```python
from build123d import *
from build123d.topology import SkipClean

# Parameters (mm, degrees)
CROQUIS1_R                 = 18
SALIENTE_EXTRUIR1_DEPTH    = 3.5
SALIENTE_EXTRUIR5_DEPTH    = 3.27
CORTAR_EXTRUIR4_REACH      = 62.83
CORTAR_EXTRUIR4_END_RADIUS = 18
CROQUIS5_W                 = 14
CROQUIS5_H                 = 0.27
CORTAR_EXTRUIR2_DEPTH      = 21
CORTAR_EXTRUIR5_DEPTH      = 10
SALIENTE_EXTRUIR6_START    = -2.2
SALIENTE_EXTRUIR6_DEPTH    = 2.2
CORTAR_EXTRUIR8_START      = 0.27
CROQUIS8_R                 = 18
CORTAR_EXTRUIR8_DEPTH      = 0.27
SALIENTE_EXTRUIR7_START    = 2.47
SALIENTE_EXTRUIR7_DEPTH    = 2.47
SALIENTE_EXTRUIR9_DEPTH    = 10
CORTAR_EXTRUIR9_START      = 10
CORTAR_EXTRUIR9_DEPTH      = 10
CROQUIS13_W                = 12.6
CROQUIS13_H                = 4.84
CROQUIS13_H_2              = 4.65
SALIENTE_EXTRUIR10_DEPTH   = 4
CROQUIS12_R                = 1
CORTAR_EXTRUIR10_DEPTH     = 18.85


with BuildPart() as part:
    # Croquis1 → Saliente-Extruir1 (new body)
    with BuildSketch(Plane.XY):
        Circle(CROQUIS1_R)
    extrude(amount=SALIENTE_EXTRUIR1_DEPTH)

    # Croquis2 → Saliente-Extruir5 (add)
    with BuildSketch(Plane.XY):
        with BuildLine():
            Line((4, 39.111635425), (4, 20.615528128))
            ThreePointArc((4, 20.615528128), (5.515132245, 20.262855582), (7, 19.798989873))
            Line((7, 19.798989873), (7, 39.928035252))
            Line((7, 39.928035252), (4, 39.928035252))
            Line((4, 39.928035252), (4, 39.111635425))
        make_face()
        with BuildLine():
            Line((-4, 20.615528128), (-4, 17.549928775))
            ThreePointArc((-4, 17.549928775), (0, 18), (4, 17.549928775))
            Line((4, 17.549928775), (4, 20.615528128))
            ThreePointArc((4, 20.615528128), (0, 21), (-4, 20.615528128))
        make_face()
        with BuildLine():
            Line((-4, 39.111635425), (-4, 20.615528128))
            ThreePointArc((-4, 20.615528128), (0, 21), (4, 20.615528128))
            Line((4, 20.615528128), (4, 39.111635425))
            Line((4, 39.111635425), (4, 39.928035252))
            Line((4, 39.928035252), (-4, 39.928035252))
            Line((-4, 39.928035252), (-4, 39.111635425))
        make_face()
        with BuildLine():
            ThreePointArc((-7, 19.798989873), (-5.515132245, 20.262855582), (-4, 20.615528128))
            Line((-4, 20.615528128), (-4, 39.111635425))
            Line((-4, 39.111635425), (-4, 39.928035252))
            Line((-4, 39.928035252), (-7, 39.928035252))
            Line((-7, 39.928035252), (-7, 19.798989873))
        make_face()
    extrude(amount=SALIENTE_EXTRUIR5_DEPTH)

    # Cortar-Extruir4: up to this cylinder (the profile starts outside it)
    with SkipClean():  # the faces are left unmerged after this step: merging them gives an invalid solid
        cortar_extruir4_end = Plane(origin=(0, 0, 0.135), z_dir=(0, 0, -1)) * Cylinder(CORTAR_EXTRUIR4_END_RADIUS, 162.66, mode=Mode.PRIVATE)
        # Croquis5 → Cortar-Extruir4 (cut, up to the surface)
        with BuildSketch(Plane(origin=(0, 40, 0), x_dir=(1, 0, 0), z_dir=(0, 1, 0)), mode=Mode.PRIVATE) as cortar_extruir4_sk1:
            with Locations((0, -0.135)):
                Rectangle(CROQUIS5_W, CROQUIS5_H)
        cortar_extruir4_tool1 = extrude(cortar_extruir4_sk1.sketch, amount=-CORTAR_EXTRUIR4_REACH, mode=Mode.PRIVATE) - cortar_extruir4_end
        add(cortar_extruir4_tool1.solids().sort_by_distance((0, 40, 0.135))[0], mode=Mode.SUBTRACT)
    add(part.part.scale(1), mode=Mode.REPLACE)  # the faces are merged on a copy

    # Croquis4 → Cortar-Extruir2 (cut)
    with BuildSketch(Plane(origin=(0, 40, 0), x_dir=(1, 0, 0), z_dir=(0, 1, 0))):
        with BuildLine():
            Line((-5.666001987, -0.685021683), (-7, -0.573296162))
            Line((-7, -0.573296162), (-7, -3.27))
            Line((-7, -3.27), (-4, -3.27))
            ThreePointArc((-4, -3.27), (-4.613533351, -1.83606535), (-5.666001987, -0.685021683))
        make_face()
        with BuildLine():
            ThreePointArc((5.666001987, -0.685021683), (4.613533351, -1.83606535), (4, -3.27))
            Line((4, -3.27), (7, -3.27))
            Line((7, -3.27), (7, -0.573296162))
            Line((7, -0.573296162), (5.666001987, -0.685021683))
        make_face()
    extrude(amount=-CORTAR_EXTRUIR2_DEPTH, mode=Mode.SUBTRACT)

    # Croquis6 → Cortar-Extruir5 (cut)
    with BuildSketch(Plane.XY):
        with BuildLine():
            ThreePointArc((-3.277147796, 5.321917166), (0, -6.25), (3.277147796, 5.321917166))
            ThreePointArc((3.277147796, 5.321917166), (2.956843582, 5.638101589), (2.807637471, 6.062724851))
            ThreePointArc((2.807637471, 6.062724851), (0, 8.575), (-2.807637471, 6.062724851))
            ThreePointArc((-2.807637471, 6.062724851), (-2.956843582, 5.638101589), (-3.277147796, 5.321917166))
        make_face()
    extrude(amount=CORTAR_EXTRUIR5_DEPTH, mode=Mode.SUBTRACT)

    # Croquis7 → Saliente-Extruir6 (add)
    with SkipClean():  # the faces are left unmerged after this step: merging them gives an invalid solid
        with BuildSketch(Plane.XY.offset(SALIENTE_EXTRUIR6_START)):
            with BuildLine():
                ThreePointArc((-5.596720258, 7.364728261), (0, -9.25), (5.596720258, 7.364728261))
                ThreePointArc((5.596720258, 7.364728261), (0, 11.575), (-5.596720258, 7.364728261))
            make_face()
            with BuildLine():
                ThreePointArc((-3.277147796, 5.321917166), (0, -6.25), (3.277147796, 5.321917166))
                ThreePointArc((3.277147796, 5.321917166), (2.956843582, 5.638101589), (2.807637471, 6.062724851))
                ThreePointArc((2.807637471, 6.062724851), (0, 8.575), (-2.807637471, 6.062724851))
                ThreePointArc((-2.807637471, 6.062724851), (-2.956843582, 5.638101589), (-3.277147796, 5.321917166))
            make_face(mode=Mode.SUBTRACT)
        extrude(amount=SALIENTE_EXTRUIR6_DEPTH)

    # Croquis8 → Cortar-Extruir8 (cut)
    with BuildSketch(Plane(origin=(0, 0, 0.27), x_dir=(-1, 0, 0), z_dir=(0, 0, -1)).offset(CORTAR_EXTRUIR8_START)):
        with Locations(Location((0, 0, 0), (0, 0, 77.160411593))):
            Circle(CROQUIS8_R)
        with BuildLine():
            ThreePointArc((-5.596720258, 7.364728261), (0, -9.25), (5.596720258, 7.364728261))
            ThreePointArc((5.596720258, 7.364728261), (0, 11.575), (-5.596720258, 7.364728261))
        make_face(mode=Mode.SUBTRACT)
    extrude(amount=-CORTAR_EXTRUIR8_DEPTH, mode=Mode.SUBTRACT)

    # Croquis9 → Saliente-Extruir7 (add)
    with BuildSketch(Plane(origin=(0, 0, 0.27), x_dir=(-1, 0, 0), z_dir=(0, 0, -1)).offset(SALIENTE_EXTRUIR7_START)):
        with BuildLine():
            Line((-7.9, -4.81170448), (-7.9, -12.127391994))
            Line((-7.9, -12.127391994), (7.9, -12.127391994))
            Line((7.9, -12.127391994), (7.9, -4.81170448))
            ThreePointArc((7.9, -4.81170448), (0, -9.25), (-7.9, -4.81170448))
        make_face()
        with BuildLine():
            Line((-7.9, 22.672608006), (-7.9, 4.81170448))
            ThreePointArc((-7.9, 4.81170448), (-6.868030798, 6.196180514), (-5.596720258, 7.364728261))
            ThreePointArc((-5.596720258, 7.364728261), (0, 11.575), (5.596720258, 7.364728261))
            ThreePointArc((5.596720258, 7.364728261), (6.868030798, 6.196180514), (7.9, 4.81170448))
            Line((7.9, 4.81170448), (7.9, 22.672608006))
            Line((7.9, 22.672608006), (-7.9, 22.672608006))
        make_face()
    extrude(amount=-SALIENTE_EXTRUIR7_DEPTH)

    # Croquis10 → Saliente-Extruir9 (add)
    with BuildSketch(Plane.XY):
        Polygon((-7.9, -12.127391994), (0, -12.127391994), (7.9, -12.127391994), (7.9, -10.927391994), (7.9, 21.472608006), (7.9, 22.672608006), (-7.9, 22.672608006), (-7.9, 21.472608006), (-7.9, 5.272608006), (-7.9, -10.927391994), align=None)
        Polygon((-6.3, -6.277391994), (-6.3, 0), (-6.3, 5.272608006), (-6.3, 16.532608006), (-6.3, 19.872608006), (-6.3, 21.472608006), (6.3, 21.472608006), (6.3, 19.872608006), (6.3, 16.532608006), (6.3, -6.277391994), (6.3, -9.327391994), (6.3, -10.927391994), (0, -10.927391994), (-6.3, -10.927391994), (-6.3, -9.327391994), align=None, mode=Mode.SUBTRACT)
    extrude(amount=-SALIENTE_EXTRUIR9_DEPTH)

    # Croquis11 → Cortar-Extruir9 (cut)
    with BuildSketch(Plane(origin=(0, 0, 0.27), x_dir=(-1, 0, 0), z_dir=(0, 0, -1)).offset(CORTAR_EXTRUIR9_START)):
        with BuildLine():
            Line((7.9, 4.81170448), (7.9, -4.81170448))
            ThreePointArc((7.9, -4.81170448), (9.25, 0), (7.9, 4.81170448))
        make_face()
        with BuildLine():
            Line((-7.9, -4.81170448), (-7.9, 4.81170448))
            ThreePointArc((-7.9, 4.81170448), (-9.25, 0), (-7.9, -4.81170448))
        make_face()
    extrude(amount=-CORTAR_EXTRUIR9_DEPTH, mode=Mode.SUBTRACT)

    # Croquis13 → Saliente-Extruir10 (add)
    with BuildSketch(Plane.XY):
        with Locations((0, 19.052608006)):
            Rectangle(CROQUIS13_W, CROQUIS13_H)
        with Locations((0, -8.602391994)):
            Rectangle(CROQUIS13_W, CROQUIS13_H_2)
    extrude(amount=-SALIENTE_EXTRUIR10_DEPTH)

    # Croquis12 → Cortar-Extruir10 (cut)
    with BuildSketch(Plane(origin=(0, 0, 0.27), x_dir=(-1, 0, 0), z_dir=(0, 0, -1))):
        with Locations(Location((0, 18.832608006, 0), (0, 0, 180))):
            Circle(CROQUIS12_R)
        with Locations(Location((0, -8.287391994, 0), (0, 0, 180))):
            Circle(CROQUIS12_R)
    extrude(amount=CORTAR_EXTRUIR10_DEPTH, mode=Mode.SUBTRACT)


solid = part.part
```
Here's how the part is built. I have some questions about the finished solid (model axes, mm). A direction names the side the tool comes from. Coordinates: 2 decimals unless noted, no trailing zeros. Order: outer loops, then holes, each group sorted by start corner. A loop starts at its lowest first (then second) coordinate and runs counter-clockwise, first axis right, second up. Notation, with made-up numbers: (73, 67) - (122, 67) arc R7 ccw to (122, 79) - close; hole circle Ø10 at (-36.75, -22). An arc over 180 degrees is marked (long way). One line per question, with ' | ' between items. Start each with the question number.
1. If we section it at D-D (y = 24): Write out the boundary of the cut face in (x, z), and give its area (3 significant figures).
2. If we section it at A-A (y = 0): Write out the boundary of the cut face in (x, z), and give its area (3 significant figures).
3. If we section it at C-C (z = -6.5): Write out the boundary of the cut face in (x, y), and give its area (3 significant figures).
4. If we mould it in two halves opening along Y, with no side actions, what happens to faces 4 (the flat face through (-6.32, 30, 0.63)), 5 (the cylindrical face through (-0.22, -7.31, -1.84))? For each: released by +Y, released by -Y, zero draft, split by the parting line, or undercut.
5. Please list where these lines run through material, in increasing order: line 1 along Y through (x, z) = (0, -0.15) (3 decimals); line 2 along X through (y, z) = (0, 1.75); line 3 along X through (y, z) = (20, -6.25). Write a range as [from, to].
6. Which directions (+Z, -Z, +X, -X, +Y, -Y) give clear straight access to the entire face, cutting with the end or side of a thin tool? Please do faces 1 (the flat face through (0, 31, 0.27)), 2 (the flat face through (0, 16.633, -3)), 3 (the cylindrical face through (0.058, 8.574, 0.61)).
7. I'm going to push flat-ended pins straight in: pin 1 Ø2.5 at (y, z) = (12, -7.5) entering from +X; pin 2 Ø3 at (x, z) = (1.5, -4) entering from -Y; pin 3 Ø11 at (x, y) = (-2, 33) entering from -Z; pin 4 Ø10.5 at (x, y) = (5, -3.5) entering from -Z. Where does each tip first touch, or does it pass through?
Model answer:
1) outline: (-7, 0.27) - (7, 0.27) - (7, 0.57) - (5.67, 0.69) arc R4.66 cw to (4, 3.27) - (-4, 3.27) arc R4.66 cw to (-5.67, 0.69) - (-7, 0.57) - close | area: 29.6 mm²
2) outline: (-18, 0.27) - (-7.9, 0.27) - (-7.9, -10) - (-6.3, -10) - (-6.3, -2.2) - (-6.25, -2.2) - (-6.25, 3.5) - (-18, 3.5) - close; (6.25, -2.2) - (6.3, -2.2) - (6.3, -10) - (7.9, -10) - (7.9, 0.27) - (18, 0.27) - (18, 3.5) - (6.25, 3.5) - close | area: 109 mm²
3) outline: (-7.9, -12.13) - (7.9, -12.13) - (7.9, 22.67) - (-7.9, 22.67) - close; hole (-6.3, -10.93) - (6.3, -10.93) - (6.3, 21.47) - (-6.3, 21.47) - close | area: 142 mm²
4) face 4: zero draft | face 5: undercut
5) line 1: y = [-12.127, -9.287], [-7.287, -6.25], [8.575, 17.833], [19.833, 22.673] | line 2: x = [-18, -6.25], [6.25, 18] | line 3: x = [-7.9, -6.3], [6.3, 7.9]
6) face 1: -Z, +X, -X, +Y | face 2: -Z | face 3: +Z, -Z
7) pin 1: stops at x = 7.9 | pin 2: stops at y = -12.13 | pin 3: stops at z = 0.27 | pin 4: stops at z = -10
